from build123d import *

# Parameters (mm, degrees)
SALIENTE_EXTRUIR1_DEPTH = 10


with BuildPart() as part:
    # Croquis1 → Saliente-Extruir1 (new body)
    with BuildSketch(Plane.XY):
        with BuildLine():
            Line((-33.5, -38.1), (33.5, -38.1))
            ThreePointArc((33.5, -38.1), (54.713203436, -29.313203436), (63.5, -8.1))
            Line((63.5, -8.1), (63.5, 8.1))
            ThreePointArc((63.5, 8.1), (54.713203436, 29.313203436), (33.5, 38.1))
            Line((33.5, 38.1), (-33.5, 38.1))
            ThreePointArc((-33.5, 38.1), (-54.713203436, 29.313203436), (-63.5, 8.1))
            Line((-63.5, 8.1), (-63.5, -8.1))
            ThreePointArc((-63.5, -8.1), (-54.713203436, -29.313203436), (-33.5, -38.1))
        make_face()
    extrude(amount=SALIENTE_EXTRUIR1_DEPTH)

    # Barrer1: sweep along a curve in space
    with BuildLine() as barrer1_path:
        Line((0, 90, 360), (0, 0, 10))
        Line((0, 90, 360), (0, 0, 710))
    # Croquis3 → Barrer1 (sweep)
    with BuildSketch(Plane.XY.offset(10)):
        with BuildLine():
            Line((33.5, -38.1), (-33.5, -38.1))
            ThreePointArc((-33.5, -38.1), (-54.713203436, -29.313203436), (-63.5, -8.1))
            Line((-63.5, -8.1), (-63.5, 8.1))
            ThreePointArc((-63.5, 8.1), (-54.713203436, 29.313203436), (-33.5, 38.1))
            Line((-33.5, 38.1), (33.5, 38.1))
            ThreePointArc((33.5, 38.1), (54.713203436, 29.313203436), (63.5, 8.1))
            Line((63.5, 8.1), (63.5, -8.1))
            ThreePointArc((63.5, -8.1), (54.713203436, -29.313203436), (33.5, -38.1))
        make_face()
    sweep(path=barrer1_path.line, transition=Transition.RIGHT)


solid = part.part
Geometry: final body of the model. Coordinates: model frame, mm. A direction names the side the tool comes from. Coordinates: 2 decimals unless noted, no trailing zeros. Order: outer loops, then holes, each group sorted by start corner. A loop starts at its lowest first (then second) coordinate and runs counter-clockwise, first axis right, second up. Notation, with made-up numbers: M 77.5,-27 L 81.5,-27 A17 cw 81.5,0 Z; hole C -2.75,81 d7. An arc over 180 degrees is marked long. One line per question, with ' | ' between items. Start each with the question number.
Item 1: Cut plane A-A, the plane x = -14.5. Return the cut outline in (y, z).
Item 2: Set-up query: faces 1 (the cylindrical face through (54.945, 29.079, 4.93)), 2 (the flat face through (-0.47, 9.86, 523.49)), 3 (the flat face through (0.47, 81.4, 541.61)), 4 (the cylindrical face through (-54.479, 29.545, 4.93)). Return all of +Z, -Z, +X, -X, +Y, -Y with unobstructed straight access to the full face (end or side cutting, diameter ignored); none if empty.
Item 3: Ray query, probe 1 along Y at (x, z) = (23, 43.5); probe 2 along Y at (x, z) = (51, 255.5); probe 3 along X at (y, z) = (94, 466). Return the intervals inside material, ascending. Write a range as [from, to].
Item 4: Pin query (flat end, axial travel): pin 1 Ø10 at (x, z) = (6.5, 101) entering from +Y; pin 2 Ø10 at (x, z) = (34.5, 227) entering from +Y; pin 3 Ø3 at (x, z) = (0, 291) entering from -Y. Return the tip coordinate at first contact, or that it passes through.
A:
1) outline: M -38.1,0 L 38.1,0 L 38.1,10 L 128.1,360 L 33.37,728.38 L -33.37,691.62 L 51.9,360 L -38.1,10 Z
2) face 1: -Z, +X, +Y | face 2: +X, -X, -Y | face 3: +Z, +X, -X, +Y | face 4: -Z, -X, +Y
3) probe 1: y = [-29.49, 46.71] | probe 2: y = [30.66, 95.6] | probe 3: x = [-52.57, 52.57]
4) pin 1: stops at y = 62.79 | pin 2: stops at y = 95.18 | pin 3: stops at y = 33.77
